Job drawing, mm, ordinate dimensions from the low corner. One solid piece. Give positions to 0.01 mm unless a question says otherwise; leave off trailing zeros. Order: outer loops, then holes, each group sorted by start corner. A loop starts at its lowest first (then second) coordinate and runs counter-clockwise, first axis right, second up.
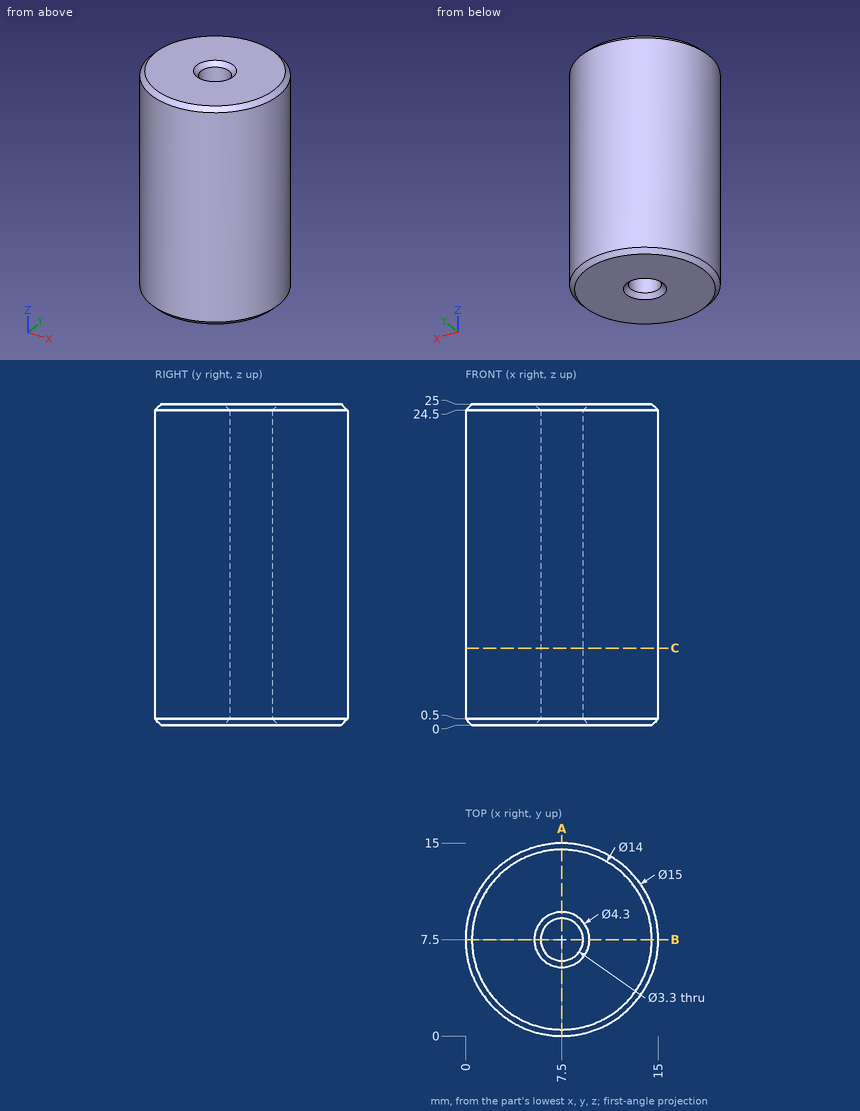
Item 1: Band-saw the part on A-A on x = 7.5. List the corners of the cut face in (y, z).
Item 2: Band-saw the part on C-C on z = 6. List the corners of the cut face in (x, y), plus the area to 3 significant figures.
Item 3: Drill centre lines: probe 1 along Y at (x, z) = (7.5, 7); probe 2 along Y at (x, z) = (9, 1.75). Where is each one in solid material? Low to high.
Item 4: Drop flat-ended pins along their axis: P1, Ø1.5, axis at x = 8.5, z = 7.5, coming from the +Y side; P2, Ø1, axis at x = 4.5, z = 16.5, coming from the -Y side; P3, Ø5, axis at y = 4.5, z = 12.5, coming from the -X side. Give the stop position or say it passes through.
Working result:
1. outline: (0, 0.5) - (0.5, 0) - (5.35, 0) - (5.85, 0.5) - (5.85, 24.5) - (5.35, 25) - (0.5, 25) - (0, 24.5) - close; (9.15, 0.5) - (9.65, 0) - (14.5, 0) - (15, 0.5) - (15, 24.5) - (14.5, 25) - (9.65, 25) - (9.15, 24.5) - close
2. outline: circle Ø15 at (7.5, 7.5); hole circle Ø3.3 at (7.5, 7.5)
2. area: 168 mm2
3. probe 1: y = 0 to 5.85, 9.15 to 15
3. probe 2: y = 0.15 to 6.81, 8.19 to 14.85
4. P1: stops at y = 15
4. P2: stops at y = 0.43
4. P3: stops at x = 0.02
